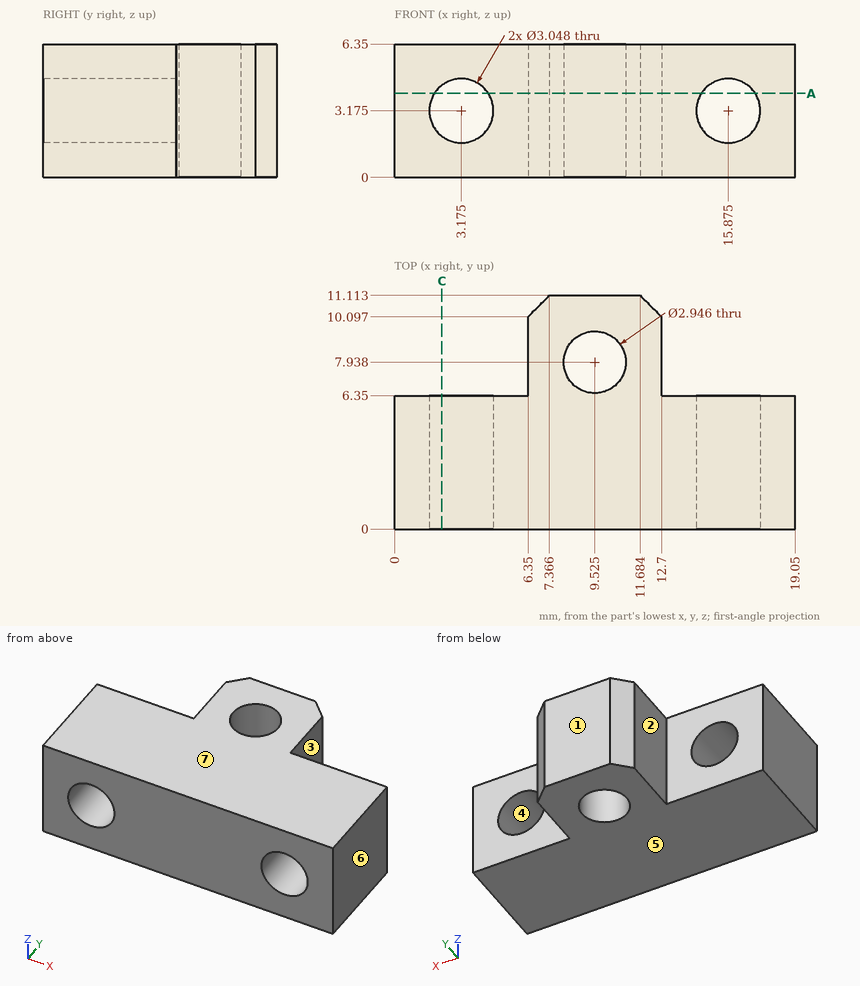
Geometry: see drawing. Coordinates: mm, zero at the bounding-box minimum. A direction names the side the tool comes from. Round coordinates to 2 decimals unless told otherwise and drop trailing zeros. Loops run counter-clockwise (first coordinate to the right, second up) from the corner with the lowest first, then second, coordinate; pieces in that order, holes last. Notation, with made-up numbers: (-26, 13) - (16, 13) arc R17 ccw to (16, 33) - close; hole circle Ø2 at (-39, 43). An arc over 180 degrees is marked (long way). Write item = value, one per line. Start each with the question number.
(1) Pull-direction query (Z, two-part tool) for the marked faces 4, 5, 6 and 7; classes: +Z half, -Z half, draft (parallel to the pull), parting line (faces both ways), or undercut.
(2) Section query C-C, the plane x = 2.25. Output: boundary loops of the cut face in (y, z).
(3) Ray query, line 1 along Y through (x, z) = (9.5, 4) (1 decimal); line 2 along X through (y, z) = (9.5, 4); line 3 along Y through (x, z) = (1, 5). Return the intervals inside material, ascending. Write a range as from..to.
(4) Section query A-A, the plane z = 4. State how many separate pieces and enclosed holes the cut face has, plus the area to 3 significant figures.
(5) Pin query (flat end, axial travel): pin 1 (2 mm diameter, centred on y = 7.5, z = 4.5, fed in from +X); pin 2 (2.5 mm diameter, centred on x = 15.875, z = 3.175, fed in from -Y); pin 3 (1.9 mm diameter, centred on x = 3.5, z = 4, fed in from +Y). Return the tip coordinate at first contact, or that it passes through.
(6) Set-up query: the marked faces 1, 2 and 3. Return all of +Z, -Z, +X, -X, +Y, -Y with unobstructed straight access to the full face (end or side cutting, diameter ignored); none if empty.
Conclusion:
q1.face_4 = undercut
q1.face_5 = -Z half
q1.face_6 = draft
q1.face_7 = +Z half
q2.outline = (0, 0) - (6.35, 0) - (6.35, 1.96) - (0, 1.96) - close; (0, 4.39) - (6.35, 4.39) - (6.35, 6.35) - (0, 6.35) - close
q3.line_1 = 0..6.5, 9.4..11.1
q3.line_2 = 6.35..12.7
q3.line_3 = 0..6.35
q4.separate_pieces = 3
q4.enclosed_holes = 1
q4.area = 111 mm2
q5.pin_1 = 12.7
q5.pin_2 = through
q5.pin_3 = 6.35
q6.face_1 = +Z, -Z, +X, -X, +Y
q6.face_2 = +Z, -Z, -X, +Y
q6.face_3 = +Z, -Z, +X, +Y
